Verification items for this drawing (mm, ordinates from the low corner). A direction names the side the tool comes from. Coordinates: 2 decimals unless noted, no trailing zeros. Order: outer loops, then holes, each group sorted by start corner. A loop starts at its lowest first (then second) coordinate and runs counter-clockwise, first axis right, second up. Notation, with made-up numbers: M 75.25,67 L 132.25,67 A19 cw 132.25,84 Z; hole C 46.25,50.5 d1. An arc over 180 degrees is marked long. One line per item, written item: value. Start each with the question number.
1) Access from +Z, -Z, +X, -X, +Y, -Y to the whole of each face (thin tool, end or side, straight path). Record for the marked faces 1, 2 and 3.
2) Draft check along Z on the marked faces 4, 5 and 6. Enter one of: pulls with the +Z half, pulls with the -Z half, needs draft (parallel to the pull), parting line crosses it, or undercut.
3) Sectioned sample at A-A, the plane x = 4. Enter the section's corners in (y, z), then the cut area to 3 significant figures.
4) Sectioned sample at D-D, the plane y = 5.25. Enter the section's corners in (x, z) (1 decimal), then the cut area to 3 significant figures.
5) Thickness scan on L1, parallel to Z at x = 2, y = 5.75; L2, parallel to X at y = 3.25, z = 7.5; L3, parallel to Z at x = 13.5, y = 3 (1 decimal). Record the ranges inside material, lowest first. Write a range as from..to.
6) Sectioned sample at C-C, the plane z = 18.25. Enter the section's corners in (x, y), then the cut area to 3 significant figures.
7) Go/stop test with flat-tipped pins: P1, Ø2, axis at y = 8, z = 13.5, coming from the -X side; P2, Ø3, axis at y = 7, z = 12, coming from the +X side; P3, Ø2, axis at x = 13, y = 3.5, coming from the +Z side. Record where each tip stops, or that it passes through.
8) Sectioned sample at B-B, the plane y = 1.25. Enter the section's corners in (x, z).
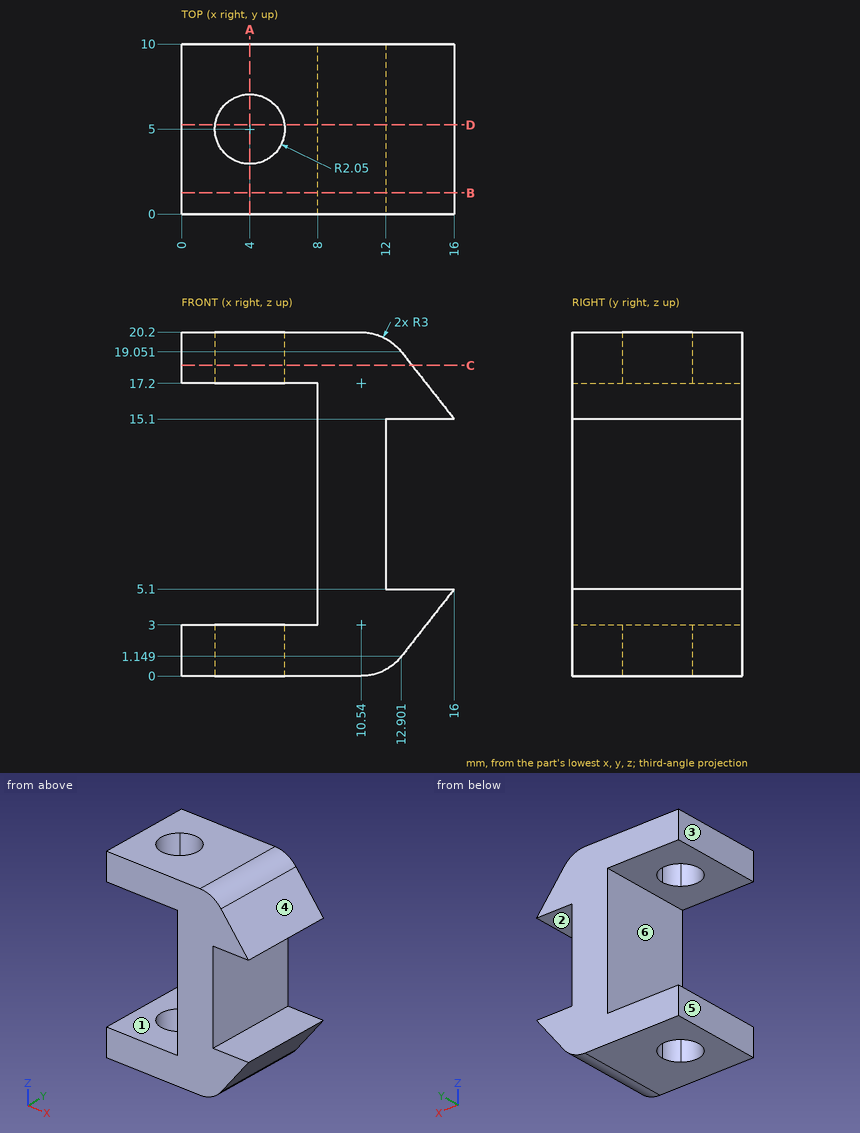
Final values:
1. face 1: -X, +Y, -Y
1. face 2: +X, +Y, -Y
1. face 3: +Z, -Z, -X, +Y, -Y
2. face 4: pulls with the +Z half
2. face 5: needs draft
2. face 6: undercut
3. outline: M 0,0 L 2.95,0 L 2.95,3 L 0,3 Z; M 0,17.2 L 2.95,17.2 L 2.95,20.2 L 0,20.2 Z; M 7.05,0 L 10,0 L 10,3 L 7.05,3 Z; M 7.05,17.2 L 10,17.2 L 10,20.2 L 7.05,20.2 Z
3. area: 35.4 mm^2
4. outline: M 0,0 L 2,0 L 2,3 L 0,3 Z; M 0,17.2 L 2,17.2 L 2,20.2 L 0,20.2 Z; M 6,0 L 10.5,0 A3 ccw 12.9,1.1 L 16,5.1 L 12,5.1 L 12,15.1 L 16,15.1 L 12.9,19.1 A3 ccw 10.5,20.2 L 6,20.2 L 6,17.2 L 8,17.2 L 8,3 L 6,3 Z
4. area: 124 mm^2
5. L1: z = 0..3, 17.2..20.2
5. L2: x = 8..12
5. L3: z = 1.9..5.1, 15.1..18.3
6. outline: M 0,0 L 13.53,0 L 13.53,10 L 0,10 Z; hole C 4,5 d4.1
6. area: 122 mm^2
7. P1: stops at x = 8
7. P2: stops at x = 12
7. P3: stops at z = 19.82
8. outline: M 0,0 L 10.54,0 A3 ccw 12.9,1.15 L 16,5.1 L 12,5.1 L 12,15.1 L 16,15.1 L 12.9,19.05 A3 ccw 10.54,20.2 L 0,20.2 L 0,17.2 L 8,17.2 L 8,3 L 0,3 Z
